```python
from build123d import *

# Parameters (mm, degrees)
BOSS_EXTRUDE1_DEPTH              = 20
CUT_EXTRUDE1_START               = -4
SKETCH2_R                        = 1.5
CUT_EXTRUDE1_DEPTH               = 25
BOSS_EXTRUDE2_DEPTH              = 23.9
SKETCH4_R                        = 3
CUT_EXTRUDE2_DEPTH               = 19
BOSS_EXTRUDE3_DEPTH              = 5
CUT_EXTRUDE3_DEPTH               = 39
CUT_EXTRUDE4_REACH               = 30.9
CUT_EXTRUDE4_OFFSET_FROM_SURFACE = 5


with BuildPart() as part:
    # Sketch1 → Boss-Extrude1 (new body)
    with BuildSketch(Plane(origin=(0, 0, 0), x_dir=(1, 0, 0), z_dir=(0, 1, 0))):
        Polygon((0, 0), (18.4, 0), (18.4, 20), (31.8, 20), (31.8, 23), (13.4, 23), (13.4, 3), (0, 3), align=None)
    extrude(amount=BOSS_EXTRUDE1_DEPTH)

    # Sketch2 → Cut-Extrude1 (cut)
    with BuildSketch(Plane.XY.offset(-20).offset(CUT_EXTRUDE1_START)):
        with Locations((25.1, 2.5)):
            Circle(SKETCH2_R)
        with Locations((25.1, 17.2)):
            Circle(SKETCH2_R)
    cut_extrude1 = extrude(amount=CUT_EXTRUDE1_DEPTH, mode=Mode.SUBTRACT)

    # Mirror1: Cut-Extrude1 across plane
    add(cut_extrude1.mirror(Plane.ZY.offset(-15.9)), mode=Mode.SUBTRACT)

    # Sketch3 → Boss-Extrude2 (add)
    with BuildSketch(Plane.ZY.offset(-13.4)):
        Polygon((-23, 0), (-23, -18), (-41, -18), (-37, 8), (-37, 20), (-23, 20), align=None)
        with BuildLine():
            Line((-33.55, -13), (-33.55, -3))
            ThreePointArc((-33.55, -3), (-31, -0.45), (-28.45, -3))
            Line((-28.45, -3), (-28.45, -13))
            ThreePointArc((-28.45, -13), (-31, -15.55), (-33.55, -13))
        make_face(mode=Mode.SUBTRACT)
    extrude(amount=-BOSS_EXTRUDE2_DEPTH)

    # Sketch4 → Cut-Extrude2 (cut, through all)
    with BuildSketch(Plane.XY.offset(-23)):
        with Locations((25.1, 2.5)):
            Circle(SKETCH4_R)
        with Locations((25.1, 17.2)):
            Circle(SKETCH4_R)
    extrude(amount=-CUT_EXTRUDE2_DEPTH, mode=Mode.SUBTRACT)

    # Sketch5 → Boss-Extrude3 (add)
    with BuildSketch(Plane.ZY.offset(-13.4)):
        Polygon((0, 0), (-23, -18), (-23, 0), align=None)
    extrude(amount=-BOSS_EXTRUDE3_DEPTH)

    # Sketch8 → Cut-Extrude3 (cut, through all)
    with BuildSketch(Plane.XZ.offset(18)):
        Polygon((37.3, -41), (36.916667761, -23), (37.3, -23), align=None)
    extrude(amount=-CUT_EXTRUDE3_DEPTH, mode=Mode.SUBTRACT)

    # Cut-Extrude4: up to this face of the body (flat: up to its plane, moved by the offset)
    cut_extrude4_end = Plane(part.part.faces().sort_by_distance((37.080777775, 1.205864864, -30.706057437))[0]).offset(-CUT_EXTRUDE4_OFFSET_FROM_SURFACE)
    # Sketch9 → Cut-Extrude4 (cut, up to the picked face)
    with BuildSketch(Plane.ZY.offset(-13.4), mode=Mode.PRIVATE) as cut_extrude4_sk1:
        with BuildLine():
            Line((-37, -3), (-37, -18))
            Line((-37, -18), (-25, -18))
            Line((-25, -18), (-25, -3))
            ThreePointArc((-25, -3), (-31, 3), (-37, -3))
        make_face()
    cut_extrude4_tool1 = split(extrude(cut_extrude4_sk1.sketch, amount=-CUT_EXTRUDE4_REACH, mode=Mode.PRIVATE), bisect_by=cut_extrude4_end, keep=Keep.BOTH, mode=Mode.PRIVATE)
    add(cut_extrude4_tool1.solids().sort_by_distance((13.4, -8.098317, -31))[0], mode=Mode.SUBTRACT)


solid = part.part
```
Input: part model. Units: mm. Frame: model coordinates. A direction names the side the tool comes from. Coordinates: 2 decimals unless noted, no trailing zeros. Loops run counter-clockwise (first coordinate to the right, second up) from the corner with the lowest first, then second, coordinate; pieces in that order, holes last. Notation, with made-up numbers: M 46,64.25 L 59,64.25 A22 cw 59,74.25 Z; hole C 10.5,-23.75 d10. An arc over 180 degrees is marked long. One line per item, written item: value.
(1) Pin query (flat end, axial travel): pin 1 (5 mm diameter, centred on y = 4, z = -36, fed in from +X); pin 2 (5.5 mm diameter, centred on x = 25.1, y = 2.5, fed in from -Z); pin 3 (4 mm diameter, centred on x = 6.7, y = 2.5, fed in from +Z); pin 4 (8 mm diameter, centred on y = -7, z = -35, fed in from -X). Return the tip coordinate at first contact, or that it passes through.
Filled in:
pin 1: x = 37.23
pin 2: z = -23
pin 3: z = 0
pin 4: x = 13.4
(2) Section C-C (y = 11). Output: boundary loops of the cut face in (x, z), and give its area (3 significant figures).
Filled in:
outline: M 0,-3 L 13.4,-3 L 13.4,-37 L 37.21,-37 L 36.92,-23 L 31.8,-23 L 31.8,-20 L 18.4,-20 L 18.4,0 L 0,0 Z
area: 527 mm^2
(3) Section D-D (x = 33.5). Output: boundary loops of the cut face in (y, z).
Filled in:
outline: M -18,-41 L 8,-37 L 20,-37 L 20,-23 L -18,-23 Z; hole M -13,-33.55 L -3,-33.55 A2.55 ccw -3,-28.45 L -13,-28.45 A2.55 ccw Z
(4) Reachability of faces 4 (the flat face through (35, -8, -33.55)), 5 (the flat face through (7, 10, -3)), 6 (the flat face through (25, 10, -20)), 7 (the cylindrical face through (21, 3, -31)) from +Z, -Z, +X, -X, +Y, -Y: full face, straight path, thin tool, end or side. Return the list, or none.
Filled in:
face 4: +X, -X
face 5: -Z, -X, +Y, -Y
face 6: +Z, +X, +Y, -Y
face 7: -X, -Y
(5) Section B-B (z = -31). Output: boundary loops of the cut face in (x, y), and give its area (3 significant figures).
Filled in:
outline: M 13.4,3 L 22.14,3 A3 cw 28.06,3 L 32.09,3 L 32.09,-0.45 L 37.09,-0.45 L 37.09,20 L 26.18,20 A3 cw long 24.02,20 L 13.4,20 Z; M 32.09,-18 L 37.09,-18 L 37.09,-15.55 L 32.09,-15.55 Z
area: 393 mm^2
(6) Pull-direction query (X, two-part tool) for faces 1 (the flat face through (23, -11, -25)), 2 (the flat face through (0, 10, -2)), 3 (the cylindrical face through (24.709, 5.474, -30.593)); classes: +X half, -X half, draft (parallel to the pull), parting line (faces both ways), or undercut.
Filled in:
face 1: draft
face 2: -X half
face 3: undercut
(7) Section A-A (x = 6.7). Output: boundary loops of the cut face in (y, z).
Filled in:
outline: M 0,-3 L 1,-3 L 1,0 L 0,0 Z; M 4,-3 L 15.7,-3 L 15.7,0 L 4,0 Z; M 18.7,-3 L 20,-3 L 20,0 L 18.7,0 Z
(8) Line query: line 1 along Y through (x, z) = (6.7, -1.35); line 2 along Z through (x, y) = (3, 18.5); line 3 along Z through (x, y) = (31, 13.5). Output: solid intervals per line, ascending. Write a range as from..to.
Filled in:
line 1: 0..1, 4..15.7, 18.7..20
line 2: -3..0
line 3: -37..-20
